Could you check a few things on this drawing? It's one solid part, dimensions in mm from its lowest x, y, z. A direction names the side the tool comes from. Give positions to 0.01 mm unless a question says otherwise; leave off trailing zeros. Order: outer loops, then holes, each group sorted by start corner. A loop starts at its lowest first (then second) coordinate and runs counter-clockwise, first axis right, second up. Notation, with made-up numbers: (20.5, -32) - (39.5, -32) arc R22 ccw to (39.5, -12) - close; hole circle Ø11 at (82, 23). An arc over 180 degrees is marked (long way). Return JSON: item names as keys, results as strings.
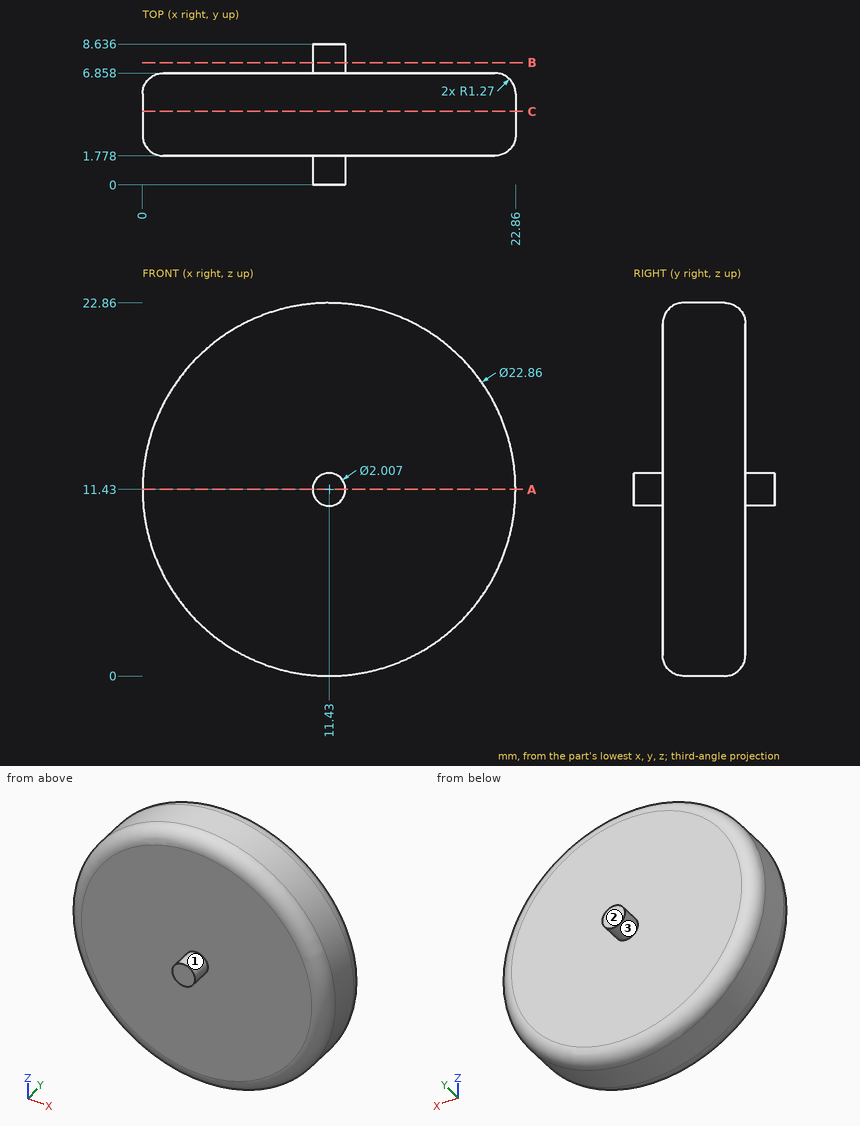
1. For pin 1 Ø4 at (x, y) = (20.5, 6.5) entering from +Z; pin 2 Ø4 at (y, z) = (2, 7.5) entering from -X; pin 3 Ø2 at (x, z) = (13.5, 20) entering from -Y; pin 4 Ø1 at (y, z) = (1, 14) entering from -X (1 decimal), each with a flat end and sliding along its axis, tell me the tip position at first contact or that it passes through.
Checks:
{"pin 1": "z = 20.29", "pin 2": "x = 0.21", "pin 3": "y = 1.78", "pin 4": "through"}
2. Suppose I cut it at C-C (y = 4.5). List the corners of the cut face in (x, z) for me, plus the area to 3 significant figures.
Checks:
{"outline": "circle Ø22.86 at (11.43, 11.43)", "area": "410 mm^2"}
3. On a 3-axis mill with a long thin cutter (end or side, diameter ignored), from which of +Z, -Z, +X, -X, +Y, -Y can I reach the whole of each face in a straight line? I mean the marked faces 1, 2 and 3. Say none if no direction works.
Checks:
{"face 1": "-Y", "face 2": "+Z, -Z, +X, -X, +Y", "face 3": "+Y"}
4. Suppose I cut it at A-A (z = 11.43). List the corners of the cut face in (x, y) for me, plus the area to 3 significant figures.
Checks:
{"outline": "(0, 3.05) arc R1.27 ccw to (1.27, 1.78) - (10.43, 1.78) - (10.43, 0) - (12.43, 0) - (12.43, 1.78) - (21.59, 1.78) arc R1.27 ccw to (22.86, 3.05) - (22.86, 5.59) arc R1.27 ccw to (21.59, 6.86) - (12.43, 6.86) - (12.43, 8.64) - (10.43, 8.64) - (10.43, 6.86) - (1.27, 6.86) arc R1.27 ccw to (0, 5.59) - close", "area": "122 mm^2"}
5. Suppose I cut it at B-B (y = 7.5). List the corners of the cut face in (x, z) for me.
Checks:
{"outline": "circle Ø2.01 at (11.43, 11.43)"}
6. If I drill on L1, parallel to Y at x = 13.75, z = 2; L2, parallel to Z at x = 12.5, y = 5.5; L3, parallel to X at y = 4.5, z = 14.75, over which ranges is the centre line in solid material (lowest first)? Write a range as [from, to].
Checks:
{"L1": "[1.78, 6.86]", "L2": "[0.05, 22.81]", "L3": "[0.49, 22.37]"}
